Verification items for this drawing (mm, ordinates from the low corner). A direction names the side the tool comes from. Coordinates: 2 decimals unless noted, no trailing zeros. Write each loop counter-clockwise with the first axis right and the second up, starting at its lowest first coordinate (ties: lowest second). Pieces come first, ordered by that corner, then holes. Notation, with made-up numbers: (-29, 23.5) -> (-8, 23.5) arc R12 ccw to (-8, 34.5) -> close; hole circle Ø11 at (75, -19.5). An arc over 180 degrees is marked (long way). Use CSV: the item, a comma, the result in double quotes.
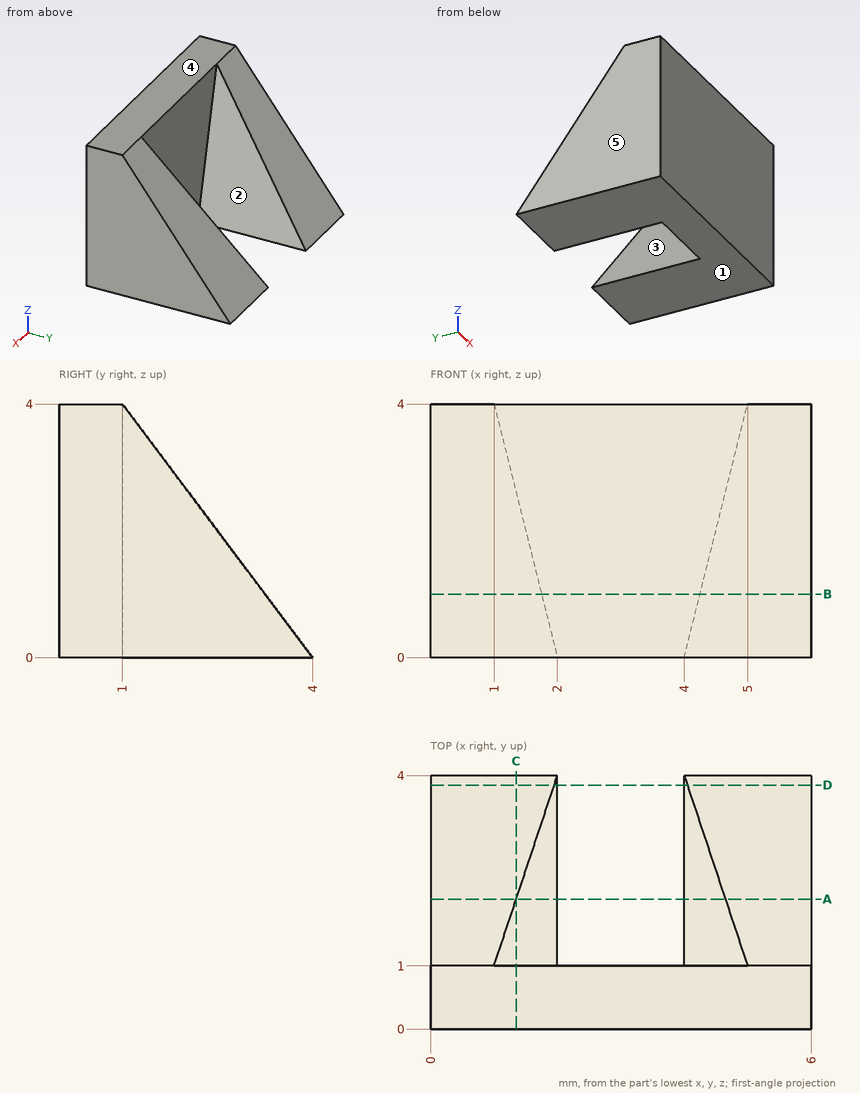
1) Gauge pin test, flat ends, axial feed: pin 1 (1 mm diameter, centred on x = 1, y = 3.5, fed in from +Z); pin 2 (1 mm diameter, centred on x = 1, z = 2, fed in from +Y) (3 decimals). Record the tip position at first contact, or that the pin passes through.
Return value:
pin 1,"z = 1.33"
pin 2,"y = 2.875"
2) Cross-section at A-A (y = 2.05). Record the boundary of the cut face in (x, z).
Return value:
outline,"(0, 0) -> (2, 0) -> (1.35, 2.6) -> (0, 2.6) -> close; (4, 0) -> (6, 0) -> (6, 2.6) -> (4.65, 2.6) -> close"
3) Set-up check for the marked faces 1 and 2: record each of +Z, -Z, +X, -X, +Y, -Y from which the full face is reachable in a straight line by a thin tool's end or side.
Return value:
face 1,"-Z, +X, -X, +Y, -Y"
face 2,"+Z, +Y"
4) Cross-section at B-B (z = 1). Record the boundary of the cut face in (x, y), plus the area to 3 significant figures.
Return value:
outline,"(0, 0) -> (6, 0) -> (6, 3.25) -> (4.25, 3.25) -> (4.25, 1) -> (1.75, 1) -> (1.75, 3.25) -> (0, 3.25) -> close"
area,"13.9 mm2"
5) Mould release check, pull along X, two halves, no side actions. Record for the marked faces 3, 4 and 5: released by +X, released by -X, zero draft, split by the parting line, or undercut.
Return value:
face 3,"undercut"
face 4,"zero draft"
face 5,"released by -X"
6) Cross-section at D-D (y = 3.85). Record the boundary of the cut face in (x, z), plus the area to 3 significant figures.
Return value:
outline,"(0, 0) -> (2, 0) -> (1.95, 0.2) -> (0, 0.2) -> close; (4, 0) -> (6, 0) -> (6, 0.2) -> (4.05, 0.2) -> close"
area,"0.790 mm2"
7) Cross-section at C-C (x = 1.35). Record the boundary of the cut face in (y, z).
Return value:
outline,"(0, 0) -> (4, 0) -> (2.05, 2.6) -> (1, 2.6) -> (1, 4) -> (0, 4) -> close"
8) Scan lines: L1, parallel to Y at x = 3.25, z = 1.3; L2, parallel to X at y = 2.75, z = 0.5 (3 decimals); L3, parallel to X at y = 1.9, z = 1.6. Record each from-to range of solid material in increasing order.
Return value:
L1,"0 to 1"
L2,"0 to 1.875, 4.125 to 6"
L3,"0 to 1.6, 4.4 to 6"
